Geometry check sheet. Reference: drawing and pictorial views, mm from the part's lowest x, y, z. A direction names the side the tool comes from. Give positions to 0.01 mm unless a question says otherwise; leave off trailing zeros. Write each loop counter-clockwise with the first axis right and the second up, starting at its lowest first coordinate (ties: lowest second). Pieces come first, ordered by that corner, then holes. Notation, with made-up numbers: (-12, 48.5) -> (-7, 48.5) arc R22 cw to (-7, 80.5) -> close; hole circle Ø7 at (-0.5, 40.5). An arc over 180 degrees is marked (long way). Return JSON: item names as keys, results as strings.
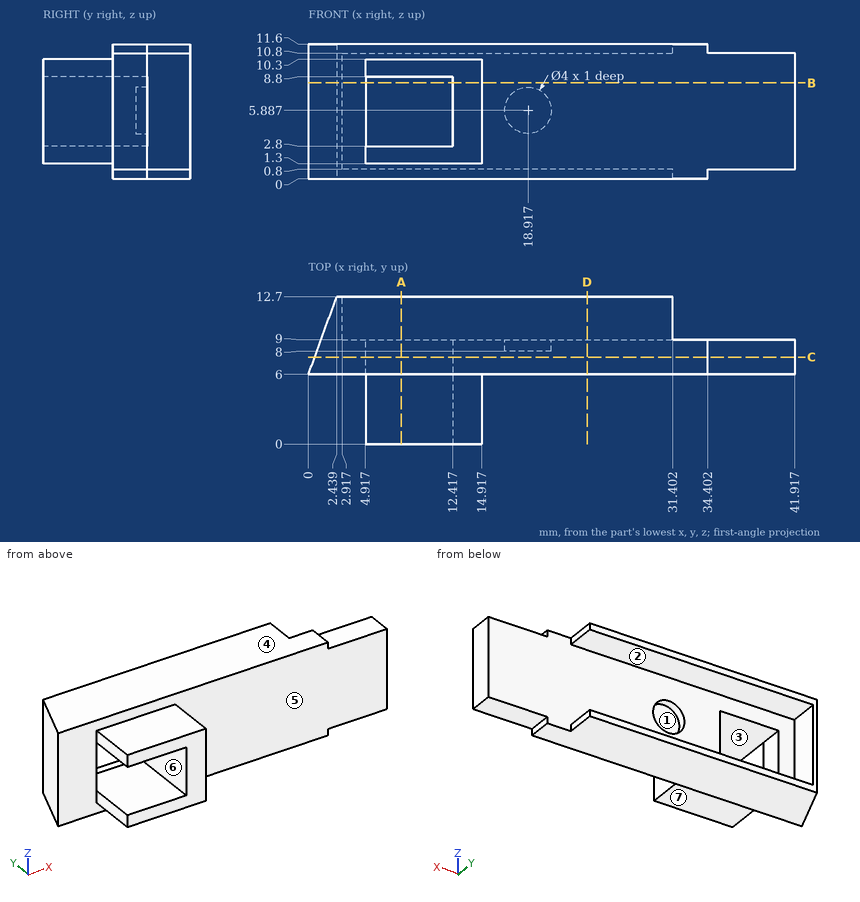
(1) Set-up check for the marked faces 1, 2 and 3: record each of +Z, -Z, +X, -X, +Y, -Y from which the full face is reachable in a straight line by a thin tool's end or side.
Reply:
{"face 1": "+Y", "face 2": "+X, +Y", "face 3": "+Y, -Y"}
(2) Cross-section at A-A on x = 8. Enter the section's corners in (y, z).
Reply:
{"outline": "(0, 1.3) -> (6, 1.3) -> (6, 0) -> (12.7, 0) -> (12.7, 0.8) -> (9, 0.8) -> (9, 2.8) -> (0, 2.8) -> close; (0, 8.8) -> (9, 8.8) -> (9, 10.8) -> (12.7, 10.8) -> (12.7, 11.6) -> (6, 11.6) -> (6, 10.3) -> (0, 10.3) -> close"}
(3) Release check for a two-part mould opening along Z. For the marked faces 4, 5, 6 and 7 record: pulls with the +Z half, pulls with the -Z half, needs draft (parallel to the pull), parting line crosses it, or undercut.
Reply:
{"face 4": "pulls with the +Z half", "face 5": "needs draft", "face 6": "undercut", "face 7": "pulls with the -Z half"}
(4) Cross-section at B-B on z = 8.25. Enter the section's corners in (x, y).
Reply:
{"outline": "(0, 6) -> (4.92, 6) -> (4.92, 9) -> (2.92, 9) -> (2.92, 12.7) -> (2.44, 12.7) -> close; (12.42, 0) -> (14.92, 0) -> (14.92, 6) -> (41.92, 6) -> (41.92, 9) -> (12.42, 9) -> close"}
(5) Cross-section at C-C on y = 7.5. Enter the section's corners in (x, z).
Reply:
{"outline": "(0.55, 0) -> (34.4, 0) -> (34.4, 0.8) -> (41.92, 0.8) -> (41.92, 10.8) -> (34.4, 10.8) -> (34.4, 11.6) -> (0.55, 11.6) -> close; hole (4.92, 2.8) -> (12.42, 2.8) -> (12.42, 8.8) -> (4.92, 8.8) -> close"}
(6) Thickness scan on L1, parallel to Z at x = 11.5, y = 8.5; L2, parallel to Z at x = 12, y = 9.25; L3, parallel to X at y = 1.75, z = 5.25. Record the ranges inside material, lowest first.
Reply:
{"L1": "0 to 2.8, 8.8 to 11.6", "L2": "0 to 0.8, 10.8 to 11.6", "L3": "12.42 to 14.92"}
(7) Cross-section at D-D on x = 24. Enter the section's corners in (y, z).
Reply:
{"outline": "(6, 0) -> (12.7, 0) -> (12.7, 0.8) -> (9, 0.8) -> (9, 10.8) -> (12.7, 10.8) -> (12.7, 11.6) -> (6, 11.6) -> close"}
(8) Depth check by flat-ended pin: pin 1 Ø5 at (x, z) = (28.5, 5) entering from -Y; pin 2 Ø3.5 at (x, z) = (29, 4) entering from +Y; pin 3 Ø2 at (x, z) = (19.5, 6) entering from +Y. Enter the tip coordinate at first touch or a pass-through.
Reply:
{"pin 1": "y = 6", "pin 2": "y = 9", "pin 3": "y = 8"}
